Autodesk Inventor part; units mm, degrees
ref_plane "YZ Plane" through (0, 0, 0) normal (1, 0, 0) x (0, 1, 0)
ref_plane "XZ Plane" through (0, 0, 0) normal (0, 1, 0) x (-1, 0, 0)
ref_plane "XY Plane" through (0, 0, 0) normal (0, 0, 1) x (1, 0, 0)
sketch "Sketch2" plane through (0, 0, 0) normal (0, 0, 1) x (1, 0, 0)
  circle A0 centre (0, 0) radius 44.5
  circle A1 centre (0, 0) radius 95
  dimension "d25" = 89
  dimension "d27" = 190
extrude "Plate2" add sketch "Sketch2" along normal blind 8
sketch "Sketch3" plane through (0, 0, 8) normal (0, 0, 1) x (1, 0, 0)
  circle A0 centre (-80, 0) radius 8.5
  circle A1 centre (0, 0) radius 80 construction
  dimension "d28" = 160
  dimension "d15" = 17
extrude "Cut1" cut sketch "Sketch3" against normal blind 8
pattern_circular "Circular Pattern1" count 4 over 360 about axis through (0, 0, -10) along (0, 0, 1) of "Cut1"
equation "\"d17\" = Thickness"
equation "\"d14\" = Thickness"
equation "\"BendReliefWidth\" = Thickness"
equation "\"BendReliefDepth\" = 0.5 * Thickness"
equation "\"CornerReliefSize\" = 4 * Thickness"
equation "\"MinimumRemnant\" = 2 * Thickness"
equation "\"TransitionRadius\" = BendRadius"
equation "\"JacobiRadiusSize\" = BendRadius"
equation "\"GapSize\" = Thickness"
properties part number "TZS 0931 FDS flange DN90" material "Steel"
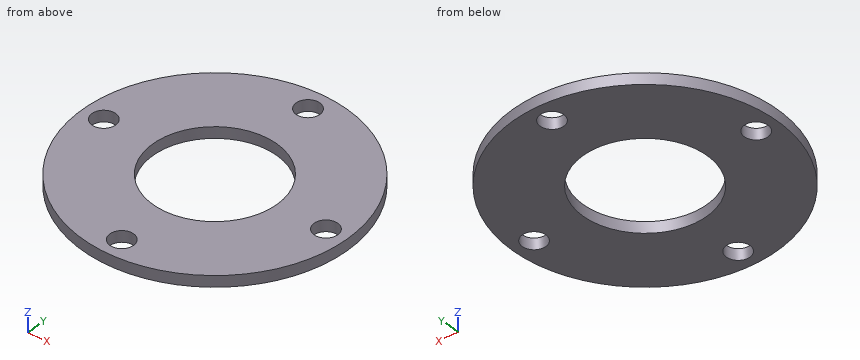
The listing builds one solid part. Answer for the finished solid, in the listing's coordinates (mm). Round coordinates to 2 decimals unless told otherwise and drop trailing zeros. Order: outer loops, then holes, each group sorted by start corner. A loop starts at its lowest first (then second) coordinate and runs counter-clockwise, first axis right, second up. Notation, with made-up numbers: (54, -23) -> (100, -23) arc R19 ccw to (100, -16) -> close; hole circle Ø9 at (-39, 87.25). An arc over 180 degrees is marked (long way). Write each question's results on one line, items separated by ' | '. Start each with the question number.
Q1. Find section D-D (x = 83). Determine the outline of the cut face in (y, z).
Q2. Each of these flat-tipped pins is pushed along its axis until it touches: pin 1 (2 mm diameter, centred on y = -31.5, z = 1.5, fed in from -X); pin 2 (1.5 mm diameter, centred on x = -39.5, z = 6, fed in from +Y). Where does it stop, or does it pass through?
Q3. Find section C-C (z = 1.75). Determine the outline of the cut face in (x, y).
Q4. Find section A-A (y = 0). Determine the outline of the cut face in (x, z), then the cut area to 3 significant figures.
Q5. Straight lines are drawn through the part: probe 1 along Y at (x, z) = (5.5, 7); probe 2 along X at (y, z) = (-41, 4); probe 3 along X at (y, z) = (33.5, 5.5). For each, find the intervals that lie inside material, in ascending order. Write a range as from..to.
Worked answers:
1) outline: (-46.22, 0) -> (-7.95, 0) -> (-7.95, 8) -> (-46.22, 8) -> close; (7.95, 0) -> (46.22, 0) -> (46.22, 8) -> (7.95, 8) -> close
2) pin 1: stops at x = -89.97 | pin 2: stops at y = 86.74
3) outline: circle Ø190 at (0, 0); hole circle Ø17 at (-80, 0); hole circle Ø89 at (0, 0); hole circle Ø17 at (0, -80); hole circle Ø17 at (0, 80); hole circle Ø17 at (80, 0)
4) outline: (-95, 0) -> (-88.5, 0) -> (-88.5, 8) -> (-95, 8) -> close; (-71.5, 0) -> (-44.5, 0) -> (-44.5, 8) -> (-71.5, 8) -> close; (44.5, 0) -> (71.5, 0) -> (71.5, 8) -> (44.5, 8) -> close; (88.5, 0) -> (95, 0) -> (95, 8) -> (88.5, 8) -> close | area: 536 mm2
5) probe 1: y = -94.84..-86.48, -73.52..-44.16, 44.16..73.52, 86.48..94.84 | probe 2: x = -85.7..-17.3, 17.3..85.7 | probe 3: x = -88.9..-29.29, 29.29..88.9
